Input: dimensioned drawing with shaded views. Units: mm. Origin: part minimum x, y, z. A direction names the side the tool comes from. Coordinates: 2 decimals unless noted, no trailing zeros. Write each loop counter-clockwise with the first axis right and the second up, starting at its lowest first coordinate (ties: lowest second). Pieces come first, ordered by that corner, then holes. Notation, with made-up numbers: (82, 88.5) - (122, 88.5) arc R26 ccw to (122, 104.5) - close; hole circle Ø1 at (-3.5, 66). An arc over 180 degrees is marked (long way). One line per question, with ' | ' between items.
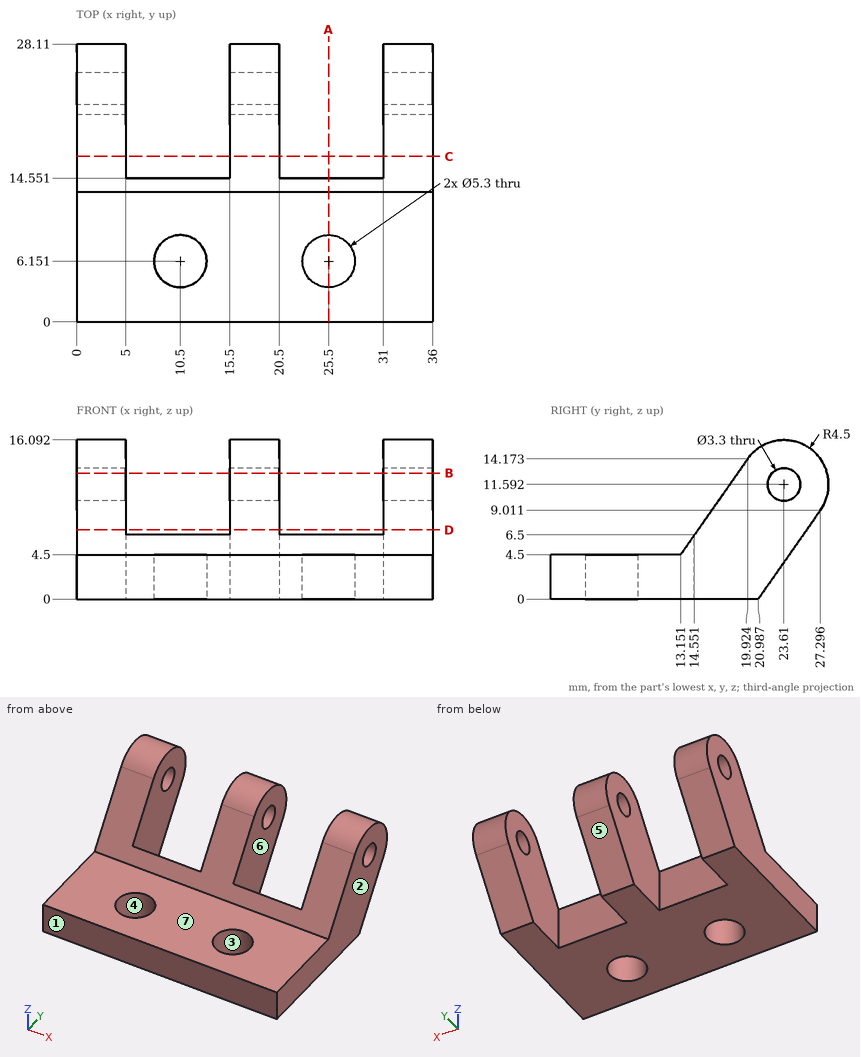
Item 1: Mould query, pull axis Y, two halves, no side actions, for the marked faces 1, 2, 3 and 4. Classes: pulls with the +Y half, pulls with the -Y half, needs draft (parallel to the pull), parting line crosses it, or undercut.
Check sheet entries:
face 1: pulls with the -Y half | face 2: needs draft | face 3: undercut | face 4: undercut
Item 2: Ray query, line 1 along X through (y, z) = (22, 12.75); line 2 along Z through (x, y) = (15.5, 10.75); line 3 along Y through (x, z) = (22.5, 1). Return the intervals inside material, ascending. Write a range as [from, to].
Check sheet entries:
line 1: [0, 5], [15.5, 20.5], [31, 36] | line 2: [0, 4.5] | line 3: [0, 14.55]
Item 3: Cut plane D-D on z = 7. Return loops of the section in (x, y).
Check sheet entries:
outline: (0, 14.9) - (5, 14.9) - (5, 25.89) - (0, 25.89) - close; (15.5, 14.9) - (20.5, 14.9) - (20.5, 25.89) - (15.5, 25.89) - close; (31, 14.9) - (36, 14.9) - (36, 25.89) - (31, 25.89) - close
Item 4: Cut plane B-B on z = 12.75. Return loops of the section in (x, y) (1 decimal), and give its area (3 significant figures).
Check sheet entries:
outline: (0, 18.9) - (5, 18.9) - (5, 22.4) - (0, 22.4) - close; (0, 24.8) - (5, 24.8) - (5, 28) - (0, 28) - close; (15.5, 18.9) - (20.5, 18.9) - (20.5, 22.4) - (15.5, 22.4) - close; (15.5, 24.8) - (20.5, 24.8) - (20.5, 28) - (15.5, 28) - close; (31, 18.9) - (36, 18.9) - (36, 22.4) - (31, 22.4) - close; (31, 24.8) - (36, 24.8) - (36, 28) - (31, 28) - close | area: 100 mm²
Item 5: Pin query (flat end, axial travel): pin 1 Ø2 at (x, z) = (8.5, 2.5) entering from +Y; pin 2 Ø6.5 at (x, y) = (27, 6) entering from +Z. Return the tip coordinate at first contact, or that it passes through.
Check sheet entries:
pin 1: y = 14.55 | pin 2: z = 4.5
Item 6: Cut plane C-C on y = 16.75. Return loops of the section in (x, z), and give its area (3 significant figures).
Check sheet entries:
outline: (0, 0) - (5, 0) - (5, 9.64) - (0, 9.64) - close; (15.5, 0) - (20.5, 0) - (20.5, 9.64) - (15.5, 9.64) - close; (31, 0) - (36, 0) - (36, 9.64) - (31, 9.64) - close | area: 145 mm²
Item 7: Access query for the marked faces 5, 6 and 7. Directions: +Z, -Z, +X, -X, +Y, -Y. A direction counts if a zero-diameter tool reaches every point of the face in a straight line with its end or side. Return the directions, or none.
Check sheet entries:
face 5: -Z, +X, -X, +Y | face 6: +Z, -Z, +Y | face 7: +Z, +X, -X, -Y
Item 8: Cut plane A-A on x = 25.5. Return loops of the section in (y, z).
Check sheet entries:
outline: (0, 0) - (3.5, 0) - (3.5, 4.5) - (0, 4.5) - close; (8.8, 0) - (14.55, 0) - (14.55, 6.5) - (13.15, 4.5) - (8.8, 4.5) - close
